Verification items for this drawing (mm, ordinates from the low corner). A direction names the side the tool comes from. Round coordinates to 2 decimals unless told otherwise and drop trailing zeros. Loops run counter-clockwise (first coordinate to the right, second up) from the corner with the lowest first, then second, coordinate; pieces in that order, holes last. Notation, with made-up numbers: (1, -18.5) -> (31, -18.5) arc R14 cw to (31, -12.5) -> close; hole circle Ø1 at (-4, 83). An arc over 180 degrees is marked (long way). One line per item, written item: value. Start each with the question number.
1. Material ranges on L1, parallel to X at y = 67.5, z = 30; L2, parallel to Z at x = 57, y = 96.5, recorded low to high.
2. Cross-section at A-A on y = 55. Record the cut outline in (x, z), then the cut area to 3 significant figures.
3. Set-up check for the marked faces 4 and 5: record each of +Z, -Z, +X, -X, +Y, -Y from which the full face is reachable in a straight line by a thin tool's end or side.
4. Go/stop test with flat-tipped pins: pin 1 (2 mm diameter, centred on y = 47.5, z = 94.5, fed in from +X); pin 2 (12 mm diameter, centred on x = 39, z = 70, fed in from +Y). Record where each tip stops, or that it passes through.
5. Release check for a two-part mould opening along X. For the marked faces 1, 2 and 3 record: +X half, -X half, draft (parallel to the pull), parting line (faces both ways), or undercut.
6. Cross-section at B-B on x = 35. Record the cut outline in (y, z), then the cut area to 3 significant figures.
7. Cross-section at C-C on z = 33.5. Record the cut outline in (x, y), then the cut area to 3 significant figures.
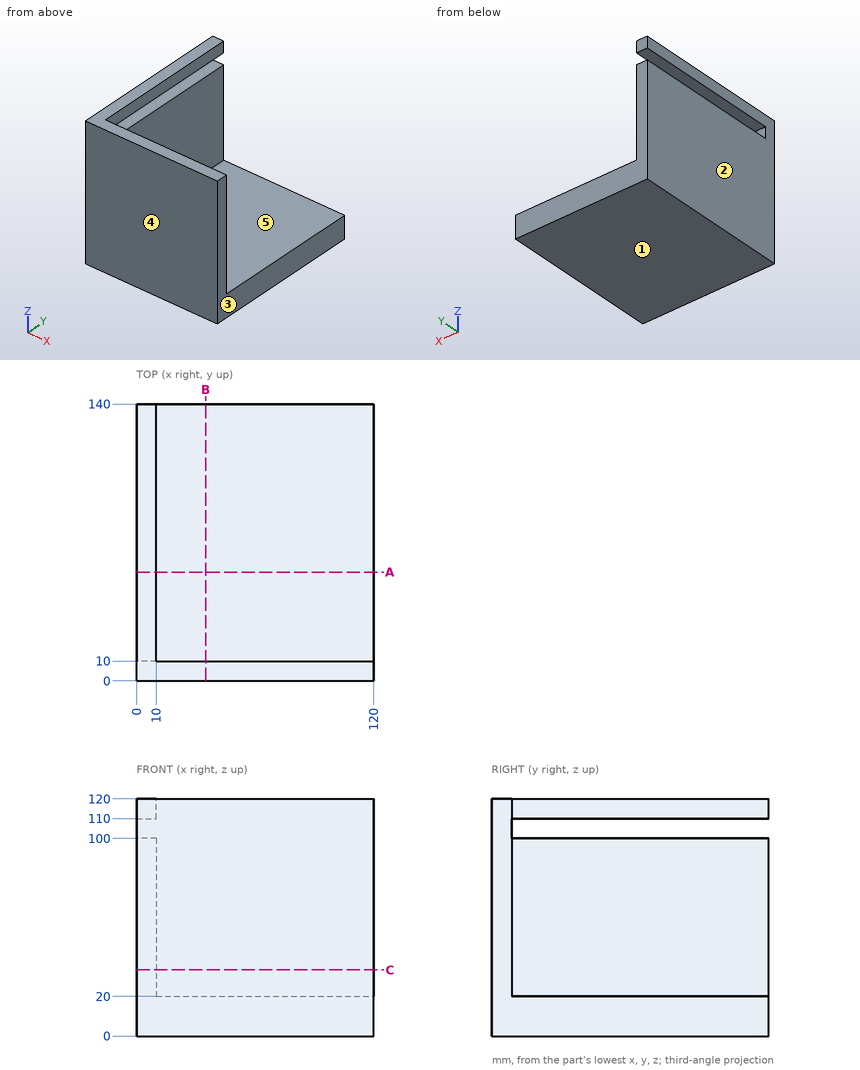
Taken from the geometry:
1. L1: x = 0 to 10
1. L2: z = 0 to 20
2. outline: (0, 0) -> (120, 0) -> (120, 20) -> (10, 20) -> (10, 100) -> (0, 100) -> close; (0, 110) -> (10, 110) -> (10, 120) -> (0, 120) -> close
2. area: 3,300 mm2
3. face 4: +Z, -Z, +X, -X, -Y
3. face 5: +Z, +X, +Y
4. pin 1: stops at x = 10
4. pin 2: stops at y = 10
5. face 1: draft
5. face 2: -X half
5. face 3: +X half
6. outline: (0, 0) -> (140, 0) -> (140, 20) -> (10, 20) -> (10, 120) -> (0, 120) -> close
6. area: 3,800 mm2
7. outline: (0, 0) -> (120, 0) -> (120, 10) -> (10, 10) -> (10, 140) -> (0, 140) -> close
7. area: 2,500 mm2
